Geometry: final body of the model. Coordinates: model frame, mm. Face numbers are marked on the shaded views. A direction names the side the tool comes from. Coordinates: 2 decimals unless noted, no trailing zeros. Write each loop counter-clockwise with the first axis right and the second up, starting at its lowest first coordinate (ties: lowest second). Pieces come first, ordered by that corner, then holes.
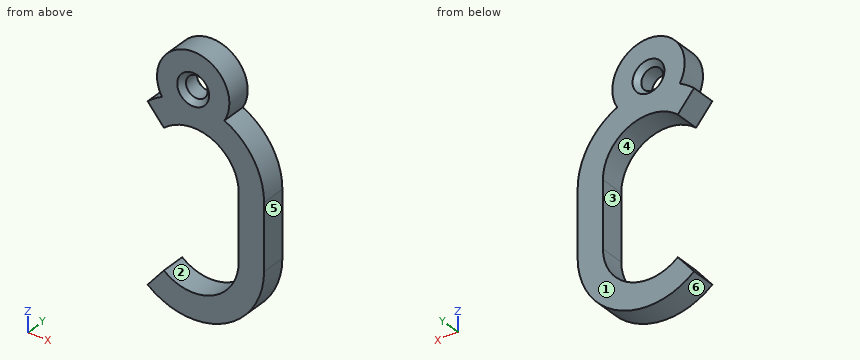
from build123d import *

# Parameters (mm, degrees)
F1_DEPTH = 2.5
F3_DEPTH = 5.001
F4_R     = 7.148228
F4_R_2   = 2.148228
F5_DEPTH = 5
F6_SIZE  = 1


with BuildPart() as f1:
    # F0 (on Front) → F1 (new body, symmetric)
    with BuildSketch(Plane.XZ):
        with BuildLine():
            Line((14, -6.5), (14, 6.5))
            ThreePointArc((14, 6.5), (0, 20.5), (-14, 6.5))
            Line((-14, 6.5), (-14, -6.5))
            ThreePointArc((-14, -6.5), (0, -20.5), (14, -6.5))
        make_face()
        with BuildLine():
            Line((9, 6.5), (9, -6.5))
            ThreePointArc((9, -6.5), (0, -15.5), (-9, -6.5))
            Line((-9, -6.5), (-9, 6.5))
            ThreePointArc((-9, 6.5), (0, 15.5), (9, 6.5))
        make_face(mode=Mode.SUBTRACT)
    extrude(amount=F1_DEPTH, both=True)

    # F2 (on face) → F3 (cut, through all)
    with BuildSketch(Plane.XZ.offset(2.5)):
        with BuildLine():
            Line((-5.785714, 13.393875), (-9, 17.223805))
            ThreePointArc((-9, 17.223805), (-12.688578, 12.41608), (-14, 6.5))
            Line((-14, 6.5), (-14, -6.5))
            ThreePointArc((-14, -6.5), (-12.688578, -12.41608), (-9, -17.223805))
            Line((-9, -17.223805), (-5.785714, -13.393875))
            ThreePointArc((-5.785714, -13.393875), (-8.156943, -10.303194), (-9, -6.5))
            Line((-9, -6.5), (-9, 6.5))
            ThreePointArc((-9, 6.5), (-8.156943, 10.303194), (-5.785714, 13.393875))
        make_face()
    extrude(amount=-F3_DEPTH, mode=Mode.SUBTRACT)

    # F4 (on face) → F5 (join, through all)
    with BuildSketch(Plane.XZ.offset(2.5)):
        with Locations((0, 22.648228)):
            Circle(F4_R)
        with Locations((0, 22.648228)):
            Circle(F4_R_2, mode=Mode.SUBTRACT)
    extrude(amount=-F5_DEPTH)

    # F6
    f6_edges = [f1.edges().sort_by_distance(p)[0] for p in [
        (2.148228, 0, 22.648228),
        (-2.148228, -2.5, 22.648228),
        (-2.148228, 2.5, 22.648228),
    ]]
    chamfer(f6_edges, length=F6_SIZE)


solid = f1.part
Item 1: Section A-A, the plane x = 0. Output: boundary loops of the cut face in (y, z), plus the area to 3 significant figures.
Derived:
outline: (-2.5, -20.5) - (2.5, -20.5) - (2.5, -15.5) - (-2.5, -15.5) - close; (-2.5, 15.5) - (2.5, 15.5) - (2.5, 19.5) - (1.5, 20.5) - (-1.5, 20.5) - (-2.5, 19.5) - close; (-2.5, 25.8) - (-1.5, 24.8) - (1.5, 24.8) - (2.5, 25.8) - (2.5, 29.8) - (-2.5, 29.8) - close
area: 73.0 mm2
Item 2: Section D-D, the plane z = -9. Output: boundary loops of the cut face in (x, y), plus the area to 3 significant figures.
Derived:
outline: (8.65, -2.5) - (13.77, -2.5) - (13.77, 2.5) - (8.65, 2.5) - close
area: 25.6 mm2
Item 3: Set-up query: the marked faces 1, 2 and 3. Return all of +Z, -Z, +X, -X, +Y, -Y with unobstructed straight access to the full face (end or side cutting, diameter ignored); none if empty.
Derived:
face 1: +Z, -Z, +X, -X, +Y
face 2: +Y, -Y
face 3: -X, +Y, -Y
Item 4: Pull-direction query (Z, two-part tool) for the marked faces 4, 5 and 6; classes: released by +Z, released by -Z, zero draft, split by the parting line, or undercut.
Derived:
face 4: undercut
face 5: zero draft
face 6: released by -Z
Item 5: Section B-B, the plane y = -0.9. Output: boundary loops of the cut face in (x, z).
Derived:
outline: (-9, -17.22) arc R14 ccw to (14, -6.5) - (14, 6.5) arc R14 ccw to (6.18, 19.06) arc R7.15 ccw (long way) to (-6.18, 19.06) arc R14 ccw to (-9, 17.22) - (-5.79, 13.39) arc R9 cw to (9, 6.5) - (9, -6.5) arc R9 cw to (-5.79, -13.39) - close; hole circle Ø4.3 at (0, 22.65)
Item 6: Pin query (flat end, axial travel): pin 1 (2 mm diameter, centred on x = 9.5, y = -0.5, fed in from +Z); pin 2 (3 mm diameter, centred on x = 2.5, y = 2, fed in from +Z); pin 3 (2 mm diameter, centred on y = -1, z = 13, fed in from -X). Return the tip coordinate at first contact, or that it passes through.
Derived:
pin 1: stops at z = 17.62
pin 2: stops at z = 29.73
pin 3: stops at x = -6.29
Item 7: Material intervals for probe 1 along Z at (x, y) = (0, 0.1); probe 2 along Z at (x, y) = (-6.5, 0.4); probe 3 along X at (y, z) = (1.7, 6), sorted ascending.
Derived:
probe 1: z = -20.5 to -15.5, 15.5 to 20.5, 24.8 to 29.8
probe 2: z = -18.9 to -14.24, 14.24 to 18.9, 19.67 to 25.62
probe 3: x = 9 to 14
Item 8: Section C-C, the plane z = 4. Output: boundary loops of the cut face in (x, y).
Derived:
outline: (9, -2.5) - (14, -2.5) - (14, 2.5) - (9, 2.5) - close
